```python
from build123d import *

# Parameters (mm, degrees)
F2_R = 2.5
F3_R = 1


with BuildPart() as f1:
    # F0 (on Front) → F1 (revolve)
    with BuildSketch(Plane.XZ):
        with BuildLine():
            add(Edge.make_bspline(
                [(0, 18.840477), (2.666021, 9.358742), (2.056838, 2.173811), (1.95, -11.159523)],
                knots=[0, 0, 0, 0, 30.063308, 30.063308, 30.063308, 30.063308], degree=3))
            Line((1.95, -11.159523), (4, -11.159523))
            Line((4, -11.159523), (4, 23.840477))
            Line((4, 23.840477), (0, 23.840477))
            Line((0, 23.840477), (0, 18.840477))
        make_face()
    revolve(axis=Axis((0, 0, 3.840477), (0, 0, 1)))

    # F2
    f2_edges = [f1.edges().sort_by_distance(p)[0] for p in [
        (-4, 0, 23.840477),
    ]]
    fillet(f2_edges, radius=F2_R)

    # F3
    f3_edges = [f1.edges().sort_by_distance(p)[0] for p in [
        (-4, 0, -11.159523),
    ]]
    fillet(f3_edges, radius=F3_R)


solid = f1.part
```
The listing builds one solid part. Answer for the finished solid, in the listing's coordinates (mm). Give positions to 0.01 mm unless a question says otherwise; leave off trailing zeros. Order: outer loops, then holes, each group sorted by start corner. A loop starts at its lowest first (then second) coordinate and runs counter-clockwise, first axis right, second up.
Item 1: Find the intervals of material crossed by probe 1 along Y at (x, z) = (0.5, 8.5); probe 2 along Y at (x, z) = (0.25, 12.5); probe 3 along X at (y, z) = (-1.25, -5), in increasing order.
From the geometry:
probe 1: y = -3.97 to -1.76, 1.76 to 3.97
probe 2: y = -3.99 to -1.35, 1.35 to 3.99
probe 3: x = -3.8 to -1.6, 1.6 to 3.8
Item 2: The part is cut by section A-A, the plane z = 21. Give the vertices of the cut face in (x, y), and give its area (3 significant figures).
From the geometry:
outline: circle Ø8 at (0, 0)
area: 50.3 mm2
Item 3: Given pin 1 Ø1.5 at (x, y) = (0, 2.5) entering from +Z; pin 2 Ø1 at (x, z) = (-2.5, 4.5) entering from +Y, each flat-ended and moving along its own axis, determine where each tip first touches the part or whether it passes through.
From the geometry:
pin 1: stops at z = 23.83
pin 2: stops at y = 3.46
